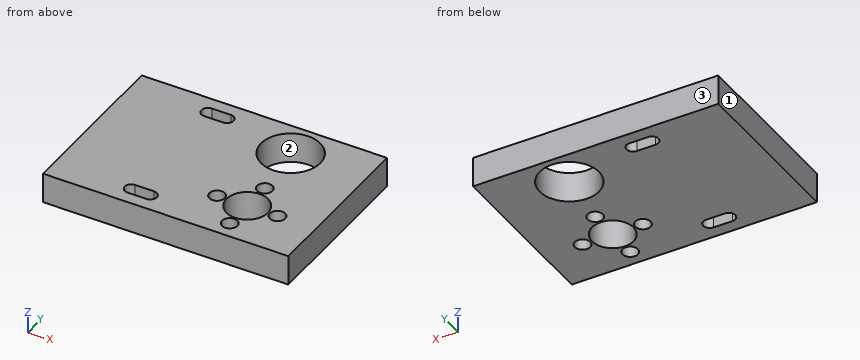
Autodesk Inventor part; units mm, degrees
ref_plane "YZ Plane" through (0, 0, 0) normal (1, 0, 0) x (0, 1, 0)
ref_plane "XZ Plane" through (0, 0, 0) normal (0, 1, 0) x (-1, 0, 0)
ref_plane "XY Plane" through (0, 0, 0) normal (0, 0, 1) x (1, 0, 0)
sketch "Sketch1" plane through (0, 0, 0) normal (0, 0, 1) x (1, 0, 0)
  line L0 (-32.5, 22.5) -> (32.5, 22.5)
  line L1 (32.5, 22.5) -> (32.5, -22.5)
  line L2 (32.5, -22.5) -> (-32.5, -22.5)
  line L3 (-32.5, -22.5) -> (-32.5, 22.5)
  point P0 (0, 0)
  point P1 (0, 22.5)
  point P2 (-32.5, 0)
  dimension "d0" = 65
  dimension "d1" = 45
extrude "Extrusion1" add sketch "Sketch1" along normal blind 8
sketch "Sketch3" plane through (0, 0, 8) normal (0, 0, 1) x (1, 0, 0)
  line L0 (-32.5, -22.5) -> (32.5, -22.5)
  line L1 (32.5, -22.5) -> (32.5, 22.5)
  line L2 (32.5, 22.5) -> (-32.5, 22.5)
  line L3 (-32.5, 22.5) -> (-32.5, -22.5)
  line L4 (-12, 17.5) -> (-7, 17.5) construction
  line L5 (-12, 15.75) -> (-7, 15.75)
  line L6 (-7, 19.25) -> (-12, 19.25)
  arc A0 (-12, 19.25) -> (-12, 15.75) centre (-12, 17.5) ccw
  arc A1 (-7, 15.75) -> (-7, 19.25) centre (-7, 17.5) ccw
  line L7 (-12, -17.5) -> (-7, -17.5) construction
  line L8 (-12, -19.25) -> (-7, -19.25)
  line L9 (-7, -15.75) -> (-12, -15.75)
  arc A2 (-12, -15.75) -> (-12, -19.25) centre (-12, -17.5) ccw
  arc A3 (-7, -19.25) -> (-7, -15.75) centre (-7, -17.5) ccw
  circle A4 centre (-9.5, -17.5) radius 1.75
  point P0 (0, 0)
  point P1 (-9.5, 17.5)
  point P2 (-9.5, -17.5)
  dimension "d8" = 5
  dimension "d9" = 3.5
  dimension "d10" = 5
  dimension "d16" = 5
  dimension "d17" = 23
  dimension "d18" = 5
  dimension "d36" = 23
extrude "Extrusion3" cut sketch "Sketch3" against normal through all contours A0 L6 A1 L5 | A2 L9 A4 L8 | A4 L9 A3 L8 | A4
sketch "Sketch4" plane through (0, 0, 8) normal (0, 0, 1) x (1, 0, 0)
  circle A0 centre (14.3605, -10) radius 11
  circle A1 centre (6.3605, -10) radius 2.05
  circle A2 centre (14.3605, -2) radius 2.05
  circle A3 centre (22.3605, -10) radius 2.05
  circle A4 centre (14.3605, -18) radius 2.05
  circle A5 centre (14.3605, -10) radius 5.5
  line L0 (32.5, -22.5) -> (32.5, 22.5)
  line L1 (-32.5, -22.5) -> (32.5, -22.5)
  dimension "d19" = 8
  dimension "d20" = 11
  dimension "d21" = 4.1
  dimension "d22" = 4.1
  dimension "d23" = 4.1
  dimension "d24" = 4.1
  dimension "d25" = 22
  dimension "d26" = 18.1395
  dimension "d27" = 8
  dimension "d28" = 8
  dimension "d29" = 8
  dimension "d30" = 12.5
extrude "Extrusion4" cut sketch "Sketch4" against normal through all contours A1 | A2 | A3 | A4 | A5
sketch "Sketch5" plane through (0, 0, 8) normal (0, 0, 1) x (1, 0, 0)
  circle A0 centre (12.5, 13) radius 7.85
  circle A1 centre (14.3605, -10) radius 5.5
  line L0 (32.5, -22.5) -> (32.5, 22.5)
  point P0 (0, 0)
  dimension "d31" = 15.7
  dimension "d32" = 23
  dimension "d33" = 20
extrude "Extrusion5" cut sketch "Sketch5" against normal blind 10 contours A0
equation "\"d18\" = d16"
properties part number "0005-10-003 Actionare seringa" material "Wood (Maple)"
Can you work these out from the model? Positions are in its coordinate system, mm. Face numbers are marked on the shaded views. Coordinates: 2 decimals unless noted, no trailing zeros. Order: outer loops, then holes, each group sorted by start corner. A loop starts at its lowest first (then second) coordinate and runs counter-clockwise, first axis right, second up. Notation, with made-up numbers: (83.5, 23) - (127.5, 23) arc R14 cw to (127.5, 29) - close; hole circle Ø8 at (50.25, 24.25). An arc over 180 degrees is marked (long way). Answer in a Markdown table with one row per item.
1. If I drill on line 1 along Y through (x, z) = (-10, 3.5); line 2 along Y through (x, z) = (13, 2.25); line 3 along Y through (x, z) = (12.5, 5.25), over which ranges is the centre line in solid material (lowest first)?
Reply:
| item | result |
|---|---|
| line 1 | y = -22.5 to -19.25, -15.75 to 15.75, 19.25 to 22.5 |
| line 2 | y = -22.5 to -19.53, -16.47 to -15.33, -4.67 to -3.53, -0.47 to 5.17, 20.83 to 22.5 |
| line 3 | y = -22.5 to -18.86, -17.14 to -15.18, -4.82 to -2.86, -1.14 to 5.15, 20.85 to 22.5 |
2. Suppose I cut it at C-C (z = 5.5). Give the number of separate pieces and of enclosed holes in the cut face, and give its area (3 significant figures).
Reply:
| item | result |
|---|---|
| separate pieces | 1 |
| enclosed holes | 8 |
| area | 2,530 mm^2 |
3. Suppose I cut it at D-D (y = -18). Please give me the cut outline in (x, z), and give its area (3 significant figures).
Reply:
| item | result |
|---|---|
| outline | (-32.5, 0) - (-13.68, 0) - (-13.68, 8) - (-32.5, 8) - close; (-5.32, 0) - (12.31, 0) - (12.31, 8) - (-5.32, 8) - close; (16.41, 0) - (32.5, 0) - (32.5, 8) - (16.41, 8) - close |
| area | 420 mm^2 |
4. Suppose I cut it at B-B (y = -10). Please give me the cut outline in (x, z), and give its area (3 significant figures).
Reply:
| item | result |
|---|---|
| outline | (-32.5, 0) - (4.31, 0) - (4.31, 8) - (-32.5, 8) - close; (8.41, 0) - (8.86, 0) - (8.86, 8) - (8.41, 8) - close; (19.86, 0) - (20.31, 0) - (20.31, 8) - (19.86, 8) - close; (24.41, 0) - (32.5, 0) - (32.5, 8) - (24.41, 8) - close |
| area | 366 mm^2 |
5. Suppose I cut it at A-A (y = -2). Please give me the cut outline in (x, z), and give its area (3 significant figures).
Reply:
| item | result |
|---|---|
| outline | (-32.5, 0) - (12.31, 0) - (12.31, 8) - (-32.5, 8) - close; (16.41, 0) - (32.5, 0) - (32.5, 8) - (16.41, 8) - close |
| area | 487 mm^2 |
6. For pin 1 (2 mm diameter, centred on x = 24, y = -6, fed in from -Z), with a flat end and sliding along its axis, tell me the tip position at first contact or that it passes through.
Reply:
| item | result |
|---|---|
| pin 1 | stops at z = 0 |
7. If we mould it in two halves opening along X, with no side actions, what happens to the marked faces 1, 2 and 3? For each: pulls with the +X half, pulls with the -X half, needs draft (parallel to the pull), parting line crosses it, or undercut.
Reply:
| item | result |
|---|---|
| face 1 | pulls with the -X half |
| face 2 | undercut |
| face 3 | needs draft |
